Here's how the part is built. I have some questions about the finished solid (model axes, mm). A direction names the side the tool comes from. Give positions to 0.01 mm unless a question says otherwise; leave off trailing zeros. Write each loop counter-clockwise with the first axis right and the second up, starting at its lowest first coordinate (ties: lowest second). Pieces come first, ordered by that corner, then holes. Notation, with made-up numbers: (12, 4.5) -> (39, 4.5) arc R16 cw to (39, 16.5) -> close; hole circle Ø11 at (71, 72.5). An arc over 180 degrees is marked (long way). Use CSV: the item, a comma, the result in double quotes. Start each with the question number.
(1) If we mould it in two halves opening along Y, with no side actions, what happens to faces 1 (the cylindrical face through (25.436, 31.177, -6.608)), 2 (the flat face through (-22.86, 5, -13)), 3 (the cylindrical face through (21.91, 12.28, -12.88))? For each: pulls with the +Y half, pulls with the -Y half, needs draft (parallel to the pull), parting line crosses it, or undercut.
(2) Suppose I cut it at A-A on z = -6.35. List the corners of the cut face in (x, y) for me, plus the area to 3 significant figures.
(3) Suppose I cut it at C-C on x = -3.5. List the corners of the cut face in (y, z) for me.
(4) For pin 1 Ø4 at (y, z) = (19, -18.5) entering from -X; pin 2 Ø6 at (x, z) = (7.5, -8.5) entering from +Y; pin 3 Ø2.5 at (y, z) = (29.21, -19.05) entering from -X; pin 4 Ø12 at (x, z) = (-11, -8.5) entering from +Y, each with a flat end and sliding along its axis, tell me the tip position at first contact or that it passes through.
(5) Which directions (+Z, -Z, +X, -X, +Y, -Y) give clear straight access to the entire face, cutting with the end or side of a thin tool? Please do faces 4 (the flat face through (0, 7, -22.86)), 5 (the flat face through (8, 10, -25.4)), 6 (the flat face through (-7, 10.16, -2)).
(6) Suppose I cut it at B-B on y = 29.21. List the corners of the cut face in (x, z) for me, plus the area to 3 significant figures.
(7) Suppose I cut it at D-D on z = -21.75. List the corners of the cut face in (x, y) for me.
(8) I need wall thicknesses on L1, parallel to Z at x = 25.5, y = 29.21; L2, parallel to Z at x = -5, y = 4; L3, parallel to Y at x = 26.2, z = -19.05. Which ranges of each line are inside material? Lowest first, please. Write a range as [from, to].
from build123d import *

# Parameters (mm, degrees)
SKETCH1_W               = 45.72
SKETCH1_H               = 25.4
BOSS_EXTRUDE1_DEPTH     = 10.16
SHELL1_T                = -2.54
SKETCH2_W               = 25.4
SKETCH2_H               = 35.56
BOSS_EXTRUDE2_DEPTH     = 5.08
FILLET1_R               = 5.08
CUT_EXTRUDE1_DEPTH      = 64.245489958
CUT_EXTRUDE1_DEPTH_BACK = 64.245489958
SKETCH3_R               = 1.984375


with BuildPart() as part:
    # Sketch1 → Boss-Extrude1 (new body)
    with BuildSketch(Plane(origin=(0, 0, 0), x_dir=(1, 0, 0), z_dir=(0, 1, 0))):
        with Locations((0, 12.7)):
            Rectangle(SKETCH1_W, SKETCH1_H)
    extrude(amount=BOSS_EXTRUDE1_DEPTH)

    # Shell1
    shell1_openings = [part.faces().sort_by_distance(p)[0] for p in [
        (0, 10.16, -12.7),
    ]]
    offset(amount=SHELL1_T, openings=shell1_openings, kind=Kind.INTERSECTION)

    # Sketch2 → Boss-Extrude2 (add)
    with BuildSketch(Plane(origin=(22.86, 0, 0), x_dir=(0, 0, -1), z_dir=(1, 0, 0))):
        with Locations((12.7, 17.78)):
            Rectangle(SKETCH2_W, SKETCH2_H)
    extrude(amount=BOSS_EXTRUDE2_DEPTH)

    # Fillet1
    # the kernel refuses this fillet: 5.08 mm, written as the material it adds along each edge
    with BuildSketch(Plane(origin=(22.86, 10.16, -25.4), x_dir=(0, 1, 0), z_dir=(0, 0, 1))) as fillet1_piece_1_section:
        with BuildLine():
            CenterArc((FILLET1_R, FILLET1_R), FILLET1_R, 180, 90)
            Line((0, FILLET1_R), (0, 0))
            Line((0, 0), (FILLET1_R, 0))
        make_face()
    fillet1_piece_1 = extrude(amount=25.4, mode=Mode.PRIVATE)
    fillet1_piece_1 = split(fillet1_piece_1, bisect_by=Plane(origin=(22.024889837, 11.456009905, -22.86), z_dir=(0, 0, -1)), keep=Keep.TOP, mode=Mode.PRIVATE)
    fillet1_piece_1 = split(fillet1_piece_1, bisect_by=Plane(origin=(20.32, 11.456009905, -24.13), z_dir=(1, 0, 0)), keep=Keep.TOP, mode=Mode.PRIVATE)
    add(fillet1_piece_1)
    with BuildSketch(Plane(origin=(22.86, 10.16, -25.4), x_dir=(0, 1, 0), z_dir=(0, 0, 1))) as fillet1_piece_2_section:
        with BuildLine():
            CenterArc((FILLET1_R, FILLET1_R), FILLET1_R, 180, 90)
            Line((0, FILLET1_R), (0, 0))
            Line((0, 0), (FILLET1_R, 0))
        make_face()
    fillet1_piece_2 = extrude(amount=25.4, mode=Mode.PRIVATE)
    fillet1_piece_2 = split(fillet1_piece_2, bisect_by=Plane(origin=(19.490686015, 10.281962579, -22.86), z_dir=(0, 0, -1)), keep=Keep.TOP, mode=Mode.PRIVATE)
    fillet1_piece_2 = split(fillet1_piece_2, bisect_by=Plane(origin=(20.32, 10.281962579, -24.13), z_dir=(-1, 0, 0)), keep=Keep.TOP, mode=Mode.PRIVATE)
    add(fillet1_piece_2)
    with BuildSketch(Plane(origin=(22.86, 10.16, -25.4), x_dir=(0, 1, 0), z_dir=(0, 0, 1))) as fillet1_piece_3_section:
        with BuildLine():
            CenterArc((FILLET1_R, FILLET1_R), FILLET1_R, 180, 90)
            Line((0, FILLET1_R), (0, 0))
            Line((0, 0), (FILLET1_R, 0))
        make_face()
    fillet1_piece_3 = extrude(amount=25.4, mode=Mode.PRIVATE)
    fillet1_piece_3 = split(fillet1_piece_3, bisect_by=Plane(origin=(22.024889837, 11.456009905, -22.86), z_dir=(0, 0, 1)), keep=Keep.TOP, mode=Mode.PRIVATE)
    fillet1_piece_3 = split(fillet1_piece_3, bisect_by=Plane(origin=(22.024889837, 11.456009905, -2.54), z_dir=(0, 0, -1)), keep=Keep.TOP, mode=Mode.PRIVATE)
    fillet1_piece_3 = split(fillet1_piece_3, bisect_by=Plane(origin=(20.32, 11.456009905, -12.7), z_dir=(1, 0, 0)), keep=Keep.TOP, mode=Mode.PRIVATE)
    add(fillet1_piece_3)
    with BuildSketch(Plane(origin=(22.86, 10.16, -25.4), x_dir=(0, 1, 0), z_dir=(0, 0, 1))) as fillet1_piece_4_section:
        with BuildLine():
            CenterArc((FILLET1_R, FILLET1_R), FILLET1_R, 180, 90)
            Line((0, FILLET1_R), (0, 0))
            Line((0, 0), (FILLET1_R, 0))
        make_face()
    fillet1_piece_4 = extrude(amount=25.4, mode=Mode.PRIVATE)
    fillet1_piece_4 = split(fillet1_piece_4, bisect_by=Plane(origin=(22.024889837, 11.456009905, -2.54), z_dir=(0, 0, 1)), keep=Keep.TOP, mode=Mode.PRIVATE)
    fillet1_piece_4 = split(fillet1_piece_4, bisect_by=Plane(origin=(20.32, 11.456009905, -1.27), z_dir=(1, 0, 0)), keep=Keep.TOP, mode=Mode.PRIVATE)
    add(fillet1_piece_4)
    with BuildSketch(Plane(origin=(22.86, 10.16, -25.4), x_dir=(0, 1, 0), z_dir=(0, 0, 1))) as fillet1_piece_5_section:
        with BuildLine():
            CenterArc((FILLET1_R, FILLET1_R), FILLET1_R, 180, 90)
            Line((0, FILLET1_R), (0, 0))
            Line((0, 0), (FILLET1_R, 0))
        make_face()
    fillet1_piece_5 = extrude(amount=25.4, mode=Mode.PRIVATE)
    fillet1_piece_5 = split(fillet1_piece_5, bisect_by=Plane(origin=(19.490686015, 10.281962579, -2.54), z_dir=(0, 0, 1)), keep=Keep.TOP, mode=Mode.PRIVATE)
    fillet1_piece_5 = split(fillet1_piece_5, bisect_by=Plane(origin=(20.32, 10.281962579, -1.27), z_dir=(-1, 0, 0)), keep=Keep.TOP, mode=Mode.PRIVATE)
    add(fillet1_piece_5)

    # Sketch3 → Cut-Extrude1 (cut, two sides: drawn at the far end of the back side and taken through both)
    with BuildSketch(Plane.ZY.offset(-22.86).offset(-CUT_EXTRUDE1_DEPTH_BACK)):
        with Locations((-19.05, 29.21)):
            Circle(SKETCH3_R)
        with Locations((-6.35, 29.21)):
            Circle(SKETCH3_R)
    extrude(amount=CUT_EXTRUDE1_DEPTH + CUT_EXTRUDE1_DEPTH_BACK, mode=Mode.SUBTRACT)


solid = part.part
Geometry says:
1,face 1,"undercut"
1,face 2,"needs draft"
1,face 3,"pulls with the +Y half"
2,outline,"(-22.86, 0) -> (27.94, 0) -> (27.94, 27.23) -> (22.86, 27.23) -> (22.86, 15.24) arc R5.08 cw to (20.32, 10.84) -> (20.32, 2.54) -> (-20.32, 2.54) -> (-20.32, 10.16) -> (-22.86, 10.16) -> close; (22.86, 31.19) -> (27.94, 31.19) -> (27.94, 35.56) -> (22.86, 35.56) -> close"
2,area,"320 mm²"
3,outline,"(0, -25.4) -> (10.16, -25.4) -> (10.16, -22.86) -> (2.54, -22.86) -> (2.54, -2.54) -> (10.16, -2.54) -> (10.16, 0) -> (0, 0) -> close"
4,pin 1,"x = 22.86"
4,pin 2,"y = 2.54"
4,pin 3,"through"
4,pin 4,"y = 10.16"
5,face 4,"+Y"
5,face 5,"-Z, +X, -X, +Y, -Y"
5,face 6,"+Z, -Z, -X, +Y"
6,outline,"(22.86, -25.4) -> (27.94, -25.4) -> (27.94, -21.03) -> (22.86, -21.03) -> close; (22.86, -17.07) -> (27.94, -17.07) -> (27.94, -8.33) -> (22.86, -8.33) -> close; (22.86, -4.37) -> (27.94, -4.37) -> (27.94, 0) -> (22.86, 0) -> close"
6,area,"88.7 mm²"
7,outline,"(-22.86, 0) -> (27.94, 0) -> (27.94, 35.56) -> (22.86, 35.56) -> (22.86, 15.24) arc R5.08 cw to (20.32, 10.84) -> (20.32, 2.54) -> (-20.32, 2.54) -> (-20.32, 10.16) -> (-22.86, 10.16) -> close"
8,L1,"[-25.4, -21.03], [-17.07, -8.33], [-4.37, 0]"
8,L2,"[-25.4, -22.86], [-2.54, 0]"
8,L3,"[0, 27.23], [31.19, 35.56]"
